```python
from build123d import *

# Parameters (mm, degrees)
F1_DEPTH  = 25.4
F2_DEPTH  = 15.24
F3_DEPTH  = 25.4
F4_DEPTH  = 10.414
F5_R      = 8.5275246161
F5_R_2    = 8.3340687874
F6_DEPTH  = 25.4
F7_R      = 6.6367792204
F8_DEPTH  = 25.4
F10_DEPTH = 63.246
F12_DEPTH = 25.4
F14_DEPTH = 25.4
F15_DEPTH = 72.644
F16_DEPTH = 3.556
F17_DEPTH = 4.572


with BuildPart() as f1:
    # F0 (on Front) → F1 (new body)
    with BuildSketch(Plane.XZ):
        Polygon((-73.6526176333, 52.2545948625), (-73.6526176333, 0), (-6.6675012931, 0), (-6.6675012931, 19.3822681904), (-58.4569200873, 19.3822681904), (-58.4569200873, 52.2545948625), align=None)
    extrude(amount=F1_DEPTH)

    # F2 (add): a face of the model
    f2_faces = [f1.faces().sort_by_distance(p)[0] for p in [
        (-47.3547272267, 0, 16.950424852),
    ]]
    extrude(f2_faces, amount=F2_DEPTH)

    # F3 (add): a face of the model
    f3_faces = [f1.faces().sort_by_distance(p)[0] for p in [
        (-6.6675012931, -5.08, 9.6911340952),
    ]]
    extrude(f3_faces, amount=F3_DEPTH)

    # F4 (add): a face of the model
    f4_faces = [f1.faces().sort_by_distance(p)[0] for p in [
        (-66.0547688603, -5.08, 52.2545948625),
    ]]
    extrude(f4_faces, amount=F4_DEPTH)

    # F5 (on face) → F6 (cut)
    with BuildSketch(Plane.XY.offset(19.3822681904)):
        with Locations((-32.3949557078, -6.2189701391)):
            Circle(F5_R)
        with Locations((-7.0090550705, -5.3727734512)):
            Circle(F5_R_2)
    extrude(amount=-F6_DEPTH, mode=Mode.SUBTRACT)

    # F7 (on face) → F8 (cut)
    with BuildSketch(Plane.YZ.offset(-58.4569200873)):
        with Locations((-6.3573834486, 35.5083160102)):
            Circle(F7_R)
    extrude(amount=-F8_DEPTH, mode=Mode.SUBTRACT)

    # F9 (on face) → F10 (cut)
    with BuildSketch(Plane.YZ.offset(-58.4569200873)):
        with BuildLine():
            Line((-12.9659945775, 62.6685948625), (-12.9659945775, 36.1191329772))
            ThreePointArc((-12.9659945775, 36.1191329772), (-7.0167461638, 42.1122602279), (0, 37.4137068119))
            Line((0, 37.4137068119), (0, 62.6685948625))
            Line((0, 62.6685948625), (-12.9659945775, 62.6685948625))
        make_face()
    extrude(amount=-F10_DEPTH, mode=Mode.SUBTRACT)

    # F11 (on face) → F12 (join)
    with BuildSketch(Plane.XY.offset(19.3822681904)):
        with BuildLine():
            ThreePointArc((18.7324987069, -13.2857691497), (16.2726896365, -20.59670587), (10.2370602665, -25.4))
            Line((10.2370602665, -25.4), (18.7324987069, -25.4))
            Line((18.7324987069, -25.4), (18.7324987069, -13.2857691497))
        make_face()
    extrude(amount=F12_DEPTH)

    # F13 (on face) → F14 (cut)
    with BuildSketch(Plane.XY.offset(19.3822681904)):
        with BuildLine():
            ThreePointArc((7.2008380666, 15.24), (14.5531964002, 8.8204791763), (18.7324987069, 0))
            Line((18.7324987069, 0), (18.7324987069, 15.24))
            Line((18.7324987069, 15.24), (7.2008380666, 15.24))
        make_face()
    extrude(amount=-F14_DEPTH, mode=Mode.SUBTRACT)

    # F15 (cut): a face of the model
    f15_faces = [f1.faces().sort_by_distance(p)[0] for p in [
        (16.4165308131, -22.484618829, 44.7822681904),
    ]]
    extrude(f15_faces, amount=-F15_DEPTH, mode=Mode.SUBTRACT)

    # F16 (cut): a face of the model
    f16_faces = [f1.faces().sort_by_distance(p)[0] for p in [
        (-66.0547688603, -19.1829972888, 62.6685948625),
    ]]
    extrude(f16_faces, amount=-F16_DEPTH, mode=Mode.SUBTRACT)

    # F17 (cut): a face of the model
    f17_faces = [f1.faces().sort_by_distance(p)[0] for p in [
        (-66.0547688603, 7.62, 62.6685948625),
    ]]
    extrude(f17_faces, amount=-F17_DEPTH, mode=Mode.SUBTRACT)


solid = f1.part
```
The model under review builds one solid part; all positions refer to its coordinate system, in mm. A direction names the side the tool comes from. Give positions to 0.01 mm unless a question says otherwise; leave off trailing zeros. Write each loop counter-clockwise with the first axis right and the second up, starting at its lowest first coordinate (ties: lowest second). Pieces come first, ordered by that corner, then holes. Notation, with made-up numbers: (34, 72) -> (55, 72) arc R7 ccw to (55, 82) -> close; hole circle Ø8 at (4, 48). An arc over 180 degrees is marked (long way). Put each result on its own line as item: value.
(1) To check wall thickness, follow probe 1 along X at (y, z) = (-0.5, 16); probe 2 along X at (y, z) = (-8.5, 27); probe 3 along Z at (x, y) = (-57, -17.5). State the ranges of each line that lie inside material, in increasing order. Write a range as from..to.
Results are:
probe 1: -73.65..-38.72, -26.07..-13.77, -0.25..18.73
probe 2: -73.65..-58.46
probe 3: 0..19.38
(2) We need section C-C, the plane x = -27.5. Give the boundary of the cut face in (y, z), and give its area (3 significant figures).
Results are:
outline: (-25.4, 0) -> (-13.2, 0) -> (-13.2, 19.38) -> (-25.4, 19.38) -> close; (0.76, 0) -> (15.24, 0) -> (15.24, 19.38) -> (0.76, 19.38) -> close
area: 517 mm²
(3) The part is to be moulded in two halves that separate along X. For faces 1 (the flat face through (-66, 8, 58.097)), 2 (the cylindrical face through (-8.09, 2.89, 9.83)), 3 (the cylindrical face through (16.335, -20.507, 9.827)), say which applies: pulls with the +X half, pulls with the -X half, needs draft (parallel to the pull), parting line crosses it, or undercut.
Results are:
face 1: needs draft
face 2: undercut
face 3: pulls with the +X half
(4) Tool access review of faces 4 (the flat face through (-66, -12.966, 48)), 5 (the flat face through (-66, -19, 59.113)), 6 (the flat face through (-20, -5, 19.382)): name each direction out of +Z, -Z, +X, -X, +Y, -Y from which nothing blocks a thin tool from reaching the whole face with its end or side.
Results are:
face 4: +Z, +X, -X
face 5: +Z, +X, -X, +Y, -Y
face 6: +Z, +X, +Y, -Y
(5) We need section A-A, the plane z = 53. Give the boundary of the cut face in (x, y), and give its area (3 significant figures).
Results are:
outline: (-73.65, -25.4) -> (-58.46, -25.4) -> (-58.46, -12.97) -> (-73.65, -12.97) -> close; (-73.65, 0) -> (-58.46, 0) -> (-58.46, 15.24) -> (-73.65, 15.24) -> close
area: 421 mm²
(6) We need section B-B, the plane y = -12. Give the boundary of the cut face in (x, z), and give its area (3 significant figures).
Results are:
outline: (-73.65, 0) -> (-38.66, 0) -> (-38.66, 19.38) -> (-58.46, 19.38) -> (-58.46, 32.01) -> (-73.65, 32.01) -> close; (-26.13, 0) -> (-12.06, 0) -> (-12.06, 19.38) -> (-26.13, 19.38) -> close; (-1.96, 0) -> (18.73, 0) -> (18.73, 19.38) -> (-1.96, 19.38) -> close
area: 1,540 mm²
(7) We need section D-D, the plane z = 6.5. Give the boundary of the cut face in (x, y).
Results are:
outline: (-73.65, -25.4) -> (10.24, -25.4) arc R13.62 ccw to (18.73, -13.29) -> (18.73, 0) arc R23.94 ccw to (7.2, 15.24) -> (-73.65, 15.24) -> close; hole circle Ø17.06 at (-32.39, -6.22); hole circle Ø16.67 at (-7.01, -5.37)
(8) For pin 1 Ø2 at (y, z) = (-11.5, 37) entering from +X; pin 2 Ø21 at (y, z) = (-6.36, 35.51) entering from +X; pin 3 Ø12 at (x, y) = (3, 7) entering from +Z; pin 4 Ø12 at (x, y) = (-65, 5) entering from +Z, all flat-tipped, find the tip position at first contact; note any pin that passes through.
Results are:
pin 1: through
pin 2: x = -58.46
pin 3: z = 19.38
pin 4: z = 58.1
